from build123d import *

# Parameters (mm, degrees)
CROQUIS1_W               = 207.5
CROQUIS1_H               = 97.5
CROQUIS1_W_2             = 204.5
CROQUIS1_H_2             = 94.5
SALIENTE_EXTRUIR1_DEPTH  = 25
CROQUIS2_W               = 207.5
CROQUIS2_H               = 97.5
SALIENTE_EXTRUIR2_DEPTH  = 3
SALIENTE_EXTRUIR3_DEPTH  = 207.5
SALIENTE_EXTRUIR4_DEPTH  = 97.5
REVOLUCI_N1_ANGLE        = 90
REVOLUCI_N2_ANGLE        = 90
REVOLUCI_N3_ANGLE        = 90
REVOLUCI_N4_ANGLE        = 90
SALIENTE_EXTRUIR5_DEPTH  = 97.5
CROQUIS10_W              = 2.5
CROQUIS10_H              = 19
SALIENTE_EXTRUIR6_DEPTH  = 204.5
CROQUIS11_W              = 2.5
CROQUIS11_H              = 19
SALIENTE_EXTRUIR7_DEPTH  = 204.5
CROQUIS13_R              = 10
SALIENTE_EXTRUIR8_DEPTH  = 0.3
CROQUIS14_R              = 10
SALIENTE_EXTRUIR9_DEPTH  = 1.5
CROQUIS15_W              = 20
CROQUIS15_H              = 20
SALIENTE_EXTRUIR10_DEPTH = 1.5
SALIENTE_EXTRUIR11_DEPTH = 1.5
CROQUIS17_R              = 10
SALIENTE_EXTRUIR12_DEPTH = 0.3
CROQUIS18_R              = 10
SALIENTE_EXTRUIR13_DEPTH = 1.5
CROQUIS19_R              = 10
SALIENTE_EXTRUIR14_DEPTH = 1.5


with BuildPart() as part:
    # Croquis1 → Saliente-Extruir1 (new body)
    with BuildSketch(Plane(origin=(0, 0, 0), x_dir=(1, 0, 0), z_dir=(0, 1, 0))):
        Rectangle(CROQUIS1_W, CROQUIS1_H)
        Rectangle(CROQUIS1_W_2, CROQUIS1_H_2, mode=Mode.SUBTRACT)
    extrude(amount=SALIENTE_EXTRUIR1_DEPTH)

    # Croquis2 → Saliente-Extruir2 (add)
    with BuildSketch(Plane(origin=(0, 25, 0), x_dir=(1, 0, 0), z_dir=(0, 1, 0))):
        Rectangle(CROQUIS2_W, CROQUIS2_H)
    extrude(amount=SALIENTE_EXTRUIR2_DEPTH)

    # Croquis3 → Saliente-Extruir3 (add)
    with BuildSketch(Plane.ZY.offset(103.75)):
        Polygon((48.75, 28), (79.533073766, -11.40053768), (78.033073766, -11.40053768), (48.75, 26.080087552), align=None)
        Polygon((-48.75, 28), (-79.533073766, -11.40053768), (-78.033073766, -11.40053768), (-48.75, 26.080087552), align=None)
    extrude(amount=-SALIENTE_EXTRUIR3_DEPTH)

    # Croquis4 → Saliente-Extruir4 (add)
    with BuildSketch(Plane.XY.offset(48.75)):
        Polygon((-103.75, 28), (-134.533073766, -11.40053768), (-133.033073766, -11.40053768), (-102.25, 28), align=None)
    extrude(amount=-SALIENTE_EXTRUIR4_DEPTH)

    # Croquis5 → Revolución1 (revolve)
    with BuildSketch(Plane.XY.offset(48.75)):
        Polygon((-103.75, 28), (-134.533073766, -11.40053768), (-133.033073766, -11.40053768), (-103.75, 26.080087552), align=None)
    revolve(axis=Axis((-103.75, 26.080087552, 48.75), (0, 1, 0)), revolution_arc=REVOLUCI_N1_ANGLE)

    # Croquis6 → Revolución2 (revolve)
    with BuildSketch(Plane.ZY.offset(103.75)):
        Polygon((-48.75, 28), (-79.533073766, -11.40053768), (-78.033073766, -11.40053768), (-48.75, 26.080087552), align=None)
    revolve(axis=Axis((-103.75, 26.080087552, -48.75), (0, 1, 0)), revolution_arc=REVOLUCI_N2_ANGLE)

    # Croquis7 → Revolución3 (revolve)
    with BuildSketch(Plane(origin=(103.75, 0, 0), x_dir=(0, 0, -1), z_dir=(1, 0, 0))):
        Polygon((48.75, 26.080087552), (48.75, 28), (79.533073766, -11.40053768), (78.033073766, -11.40053768), align=None)
    revolve(axis=Axis((103.75, 26.080087552, -48.75), (0, -1, 0)), revolution_arc=REVOLUCI_N3_ANGLE)

    # Croquis8 → Revolución4 (revolve)
    with BuildSketch(Plane(origin=(103.75, 0, 0), x_dir=(0, 0, -1), z_dir=(1, 0, 0))):
        Polygon((-48.75, 28), (-79.533073766, -11.40053768), (-78.033073766, -11.40053768), (-48.75, 26.080087552), align=None)
    revolve(axis=Axis((103.75, 26.080087552, 48.75), (0, 1, 0)), revolution_arc=REVOLUCI_N4_ANGLE)

    # Croquis9 → Saliente-Extruir5 (add)
    with BuildSketch(Plane(origin=(0, 0, 48.75), x_dir=(-1, 0, 0), z_dir=(0, 0, -1))):
        Polygon((-103.75, 28), (-103.75, 26.080087552), (-133.033073766, -11.40053768), (-134.533073766, -11.40053768), align=None)
    extrude(amount=SALIENTE_EXTRUIR5_DEPTH)

    # Croquis10 → Saliente-Extruir6 (add)
    with BuildSketch(Plane.ZY.offset(-102.25)):
        with Locations((46, 15.5)):
            Rectangle(CROQUIS10_W, CROQUIS10_H)
    extrude(amount=SALIENTE_EXTRUIR6_DEPTH)

    # Croquis11 → Saliente-Extruir7 (add)
    with BuildSketch(Plane.ZY.offset(-102.25)):
        with Locations((-46, 15.5)):
            Rectangle(CROQUIS11_W, CROQUIS11_H)
    extrude(amount=SALIENTE_EXTRUIR7_DEPTH)



with BuildPart() as body_2:
    # Croquis13 → Saliente-Extruir8 (new body)
    with BuildSketch(Plane(origin=(-102.25, 0, 0), x_dir=(0, 0, -1), z_dir=(1, 0, 0))):
        with Locations((0, -10)):
            Circle(CROQUIS13_R)
    extrude(amount=SALIENTE_EXTRUIR8_DEPTH)

    # Croquis14 → Saliente-Extruir9 (add)
    with BuildSketch(Plane.ZY.offset(102.25)):
        with Locations((0, -10)):
            Circle(CROQUIS14_R)
    extrude(amount=SALIENTE_EXTRUIR9_DEPTH)


with BuildPart() as part_1:
    add(part.part)

    add(body_2.part)  # Saliente-Extruir10 merges body 2
    # Croquis15 → Saliente-Extruir10 (add)
    with BuildSketch(Plane.ZY.offset(103.75)):
        Rectangle(CROQUIS15_W, CROQUIS15_H)
    extrude(amount=-SALIENTE_EXTRUIR10_DEPTH)

    # Croquis16 → Saliente-Extruir11 (add)
    with BuildSketch(Plane.ZY.offset(-102.25)):
        with BuildLine():
            Line((10, -10), (0, -10))
            Line((0, -10), (-10, -10))
            ThreePointArc((-10, -10), (0, -20), (10, -10))
        make_face()
        with BuildLine():
            ThreePointArc((10, -10), (7.071067812, -2.928932188), (0, 0))
            Line((0, 0), (0, -10))
            Line((0, -10), (10, -10))
        make_face()
        with BuildLine():
            Line((0, -10), (0, 0))
            ThreePointArc((0, 0), (-7.071067812, -2.928932188), (-10, -10))
            Line((-10, -10), (0, -10))
        make_face()
        with BuildLine():
            ThreePointArc((-10, -10), (-7.071067812, -2.928932188), (0, 0))
            Line((0, 0), (-10, 0))
            Line((-10, 0), (-10, -10))
        make_face()
        with BuildLine():
            Line((10, 0), (0, 0))
            ThreePointArc((0, 0), (7.071067812, -2.928932188), (10, -10))
            Line((10, -10), (10, 0))
        make_face()
        Polygon((-10, 0), (0, 0), (10, 0), (10, 10), (-10, 10), align=None)
    extrude(amount=-SALIENTE_EXTRUIR11_DEPTH)

    # Croquis17 → Saliente-Extruir12 (add)
    with BuildSketch(Plane.ZY.offset(-102.25)):
        with Locations((0, -10)):
            Circle(CROQUIS17_R)
    extrude(amount=SALIENTE_EXTRUIR12_DEPTH)

    # Croquis18 → Saliente-Extruir13 (add)
    with BuildSketch(Plane.ZY.offset(-101.95)):
        with Locations((0, -10)):
            Circle(CROQUIS18_R)
    extrude(amount=SALIENTE_EXTRUIR13_DEPTH)

    # Croquis19 → Saliente-Extruir14 (add)
    with BuildSketch(Plane(origin=(-101.95, 0, 0), x_dir=(0, 0, -1), z_dir=(1, 0, 0))):
        with Locations((0, -10)):
            Circle(CROQUIS19_R)
    extrude(amount=SALIENTE_EXTRUIR14_DEPTH)


solid = part_1.part
The model under review builds one solid part; all positions refer to its coordinate system, in mm. A direction names the side the tool comes from. Round coordinates to 2 decimals unless told otherwise and drop trailing zeros. Loops run counter-clockwise (first coordinate to the right, second up) from the corner with the lowest first, then second, coordinate; pieces in that order, holes last. Notation, with made-up numbers: (28, 65) - (70, 65) arc R11 cw to (70, 78) - close; hole circle Ø5 at (42, 65.5). An arc over 180 degrees is marked (long way). Use CSV: the item, a comma, the result in double quotes.
(1) Take a section at C-C, the plane z = -22. Give the boundary of the cut face in (x, y).
Working result:
outline,"(-134.53, -11.4) - (-133.03, -11.4) - (-103.75, 26.08) - (-103.75, 0) - (-102.25, 0) - (-102.25, 25) - (102.25, 25) - (102.25, 0) - (103.75, 0) - (103.75, 26.08) - (133.03, -11.4) - (134.53, -11.4) - (103.75, 28) - (-103.75, 28) - close"
(2) Clearance check with flat-ended pins moving along their axes: P1, Ø5, axis at x = -6, y = 4, coming from the +Z side; P2, Ø1, axis at x = 64.5, z = -40.5, coming from the -Y side; P3, Ø1, axis at x = -74.5, y = 14.5, coming from the -Z side. State where each tip first meets the part, or that it passes through.
Working result:
P1,"stops at z = 69.45"
P2,"stops at y = 25"
P3,"stops at z = -59.69"
(3) The part is to be moulded in two halves that separate along X. For faces 4 (the flat face through (-1.453, 8.576, 63.926)), 5 (the flat face through (119.36, 8.02, 0.68)), 6 (the flat face through (103.75, 14, -1)), 7 (the cylindrical face through (-101.756, -18.872, -4.614)), say which applies: pulls with the +X half, pulls with the -X half, needs draft (parallel to the pull), parting line crosses it, or undercut.
Working result:
face 4,"needs draft"
face 5,"pulls with the +X half"
face 6,"undercut"
face 7,"undercut"
(4) Machinability: for faces 1 (the conical face through (-114.7, 8, -59.9)), 2 (the flat face through (-1.453, 7.077, 63.597)), 3 (the cylindrical face through (101.756, -18.872, 4.614)), which of the approach directions +Z, -Z, +X, -X, +Y, -Y give a long, thin tool a straight path to every point of the face, cutting with its end or side? Answer none if there is none.
Working result:
face 1,"-Z, -X, +Y"
face 2,"-Y"
face 3,"none"
(5) Take a section at B-B, the plane x = -29. Give the boundary of the cut face in (y, z), plus the area to 3 significant figures.
Working result:
outline,"(-11.4, -79.53) - (28, -48.75) - (28, 48.75) - (-11.4, 79.53) - (-11.4, 78.03) - (26.08, 48.75) - (0, 48.75) - (0, 47.25) - (6, 47.25) - (6, 44.75) - (25, 44.75) - (25, -44.75) - (6, -44.75) - (6, -47.25) - (0, -47.25) - (0, -48.75) - (26.08, -48.75) - (-11.4, -78.03) - close"
area,"578 mm^2"
(6) For line 1 (Z direction, x = 87.5, y = 3); line 2 (Z direction, x = 3, y = 0.5); line 3 (X direction, y = 24, z = 40), list the stretches that pass through material, from the lowest coordinate up.
Working result:
line 1,"z = -68.28 to -66.78, -48.75 to -47.25, 47.25 to 48.75, 66.78 to 68.28"
line 2,"z = -70.24 to -68.74, -48.75 to -47.25, 47.25 to 48.75, 68.74 to 70.24"
line 3,"x = -106.88 to -105.38, -103.75 to -102.25, 102.25 to 103.75, 105.38 to 106.88"
(7) Take a section at A-A, the plane z = 0. Give the boundary of the cut face in (x, y), plus the area to 3 significant figures.
Working result:
outline,"(-134.53, -11.4) - (-133.03, -11.4) - (-103.75, 26.08) - (-103.75, -20) - (-100.45, -20) - (-100.45, 0) - (-102.25, 0) - (-102.25, 25) - (102.25, 25) - (102.25, 0) - (100.45, 0) - (100.45, -20) - (103.75, -20) - (103.75, 26.08) - (133.03, -11.4) - (134.53, -11.4) - (103.75, 28) - (-103.75, 28) - close"
area,"945 mm^2"
